Can you work these out from the drawing? Everything is in mm from the part's minimum corner. A direction names the side the tool comes from. Coordinates: 2 decimals unless noted, no trailing zeros. Loops run counter-clockwise (first coordinate to the right, second up) from the corner with the lowest first, then second, coordinate; pieces in that order, holes last.
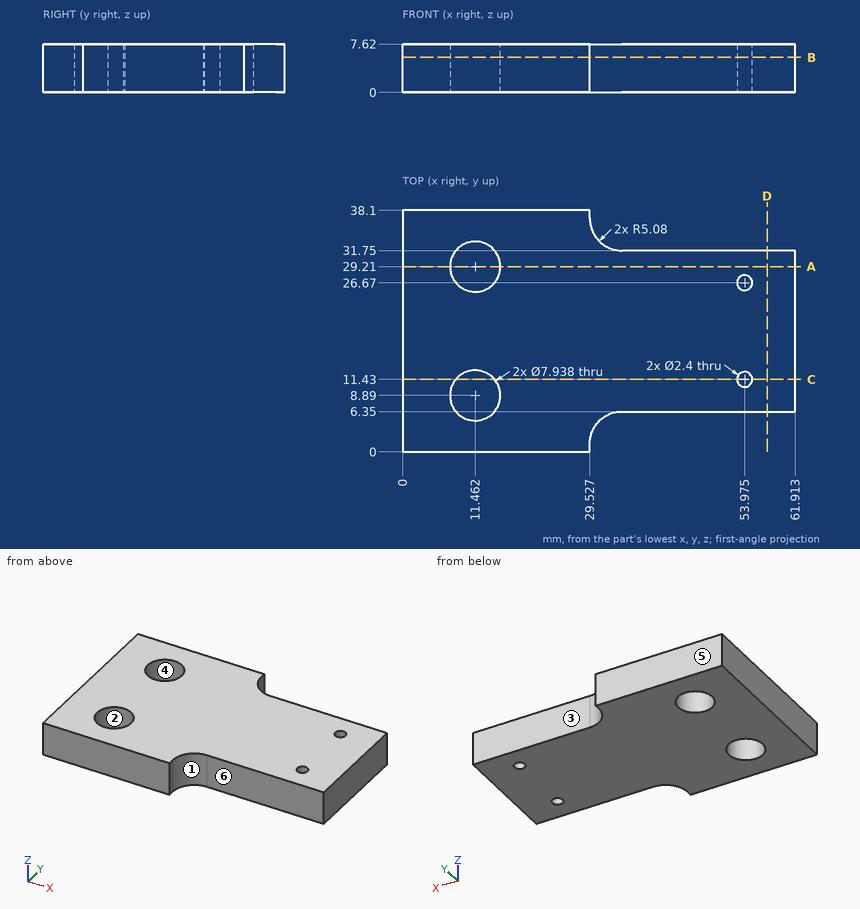
Item 1: Suppose I cut it at A-A, the plane y = 29.21. Please give me the cut outline in (x, z).
Results are:
outline: (0, 0) - (7.49, 0) - (7.49, 7.62) - (0, 7.62) - close; (15.43, 0) - (61.91, 0) - (61.91, 7.62) - (15.43, 7.62) - close
Item 2: Suppose I cut it at D-D, the plane x = 57.5. Please give me the cut outline in (y, z).
Results are:
outline: (6.35, 0) - (31.75, 0) - (31.75, 7.62) - (6.35, 7.62) - close
Item 3: Suppose I cut it at B-B, the plane z = 5.5. Count the separate pieces of the cut face and the enclosed holes in it, plus the area to 3 significant figures.
Results are:
separate pieces: 1
enclosed holes: 4
area: 1,850 mm2
Item 4: Suppose I cut it at C-C, the plane y = 11.43. Please give me the cut outline in (x, z) (1 decimal), plus the area to 3 significant figures.
Results are:
outline: (0, 0) - (8.4, 0) - (8.4, 7.6) - (0, 7.6) - close; (14.5, 0) - (52.8, 0) - (52.8, 7.6) - (14.5, 7.6) - close; (55.2, 0) - (61.9, 0) - (61.9, 7.6) - (55.2, 7.6) - close
area: 407 mm2
Item 5: We'd pull the mould along X, two halves only. Please class the marked faces 1, 2, 3 and 4: +X half, -X half, draft (parallel to the pull), parting line (faces both ways), or undercut.
Results are:
face 1: +X half
face 2: undercut
face 3: draft
face 4: undercut
Item 6: On a 3-axis mill with a long thin cutter (end or side, diameter ignored), from which of +Z, -Z, +X, -X, +Y, -Y can I reach the whole of each face in a straight line? I mean the marked faces 5 and 6. Say none if no direction works.
Results are:
face 5: +Z, -Z, +X, -X, +Y
face 6: +Z, -Z, +X, -Y
Item 7: I'm going to push flat-ended pins straight in: P1, Ø1, axis at y = 0.5, z = 3.5, coming from the +X side; P2, Ø1, axis at x = 34.5, z = 1.5, coming from the -Y side; P3, Ø1.5, axis at x = 36.5, z = 6.5, coming from the +Y side. Where does each tip first touch, or does it pass through?
Results are:
P1: stops at x = 29.53
P2: stops at y = 6.31
P3: stops at y = 31.75
Item 8: I need wall thicknesses on line 1 along X through (y, z) = (10.5, 4) (1 decimal); line 2 along Y through (x, z) = (53, 7); line 3 along Y through (x, z) = (48.5, 6). Which ranges of each line are inside material? Lowest first, please.
Results are:
line 1: x = 0 to 7.8, 15.1 to 53.2, 54.7 to 61.9
line 2: y = 6.35 to 10.73, 12.13 to 25.97, 27.37 to 31.75
line 3: y = 6.35 to 31.75
